Job drawing, mm, ordinate dimensions from the low corner. One solid piece. A direction names the side the tool comes from. Give positions to 0.01 mm unless a question says otherwise; leave off trailing zeros. Loops run counter-clockwise (first coordinate to the right, second up) from the corner with the lowest first, then second, coordinate; pieces in that order, holes last. Notation, with made-up numbers: (42, -26.5) - (70, -26.5) arc R15 ccw to (70, -1.5) - close; hole circle Ø1 at (26.5, 35). An arc over 180 degrees is marked (long way). Answer as CSV lines item,"result". Start each with the question number.
Item 1: Saw through at D-D on x = 18. Give the cut face in (y, z).
Item 2: Saw through at A-A on x = 120. Give the cut face in (y, z).
Item 3: Tool access for the marked faces 1, 2 and 3: list every direction of +Z, -Z, +X, -X, +Y, -Y with a clear straight run to the whole face (end or side of a thin tool).
Item 4: Drill centre lines: L1, parallel to Y at x = 120, z = 38.5; L2, parallel to Y at x = 120, z = 33.5; L3, parallel to Z at x = 220, y = 138. Where is each one in solid material? Low to high. Write a range as from..to.
Item 5: Pin check, flat tips, straight feed: pin 1 (12 mm diameter, centred on y = 66, z = 12.5, fed in from -X); pin 2 (4 mm diameter, centred on y = 175.5, z = 40.5, fed in from +X); pin 3 (2 mm diameter, centred on x = 121.5, y = 207, fed in from +Z). Stop position of each tip, or through.
Item 6: Pull direction Y, two halves, no side cores. Call the marked faces 4, 5 and 6: pulls with the +Y half, pulls with the -Y half, needs draft (parallel to the pull), parting line crosses it, or undercut.
Item 7: Saw through at B-B on y = 120. Give the cut face in (x, z), plus the area to 3 significant figures.
Item 8: Saw through at C-C on z = 39. Give the cut face in (x, y).
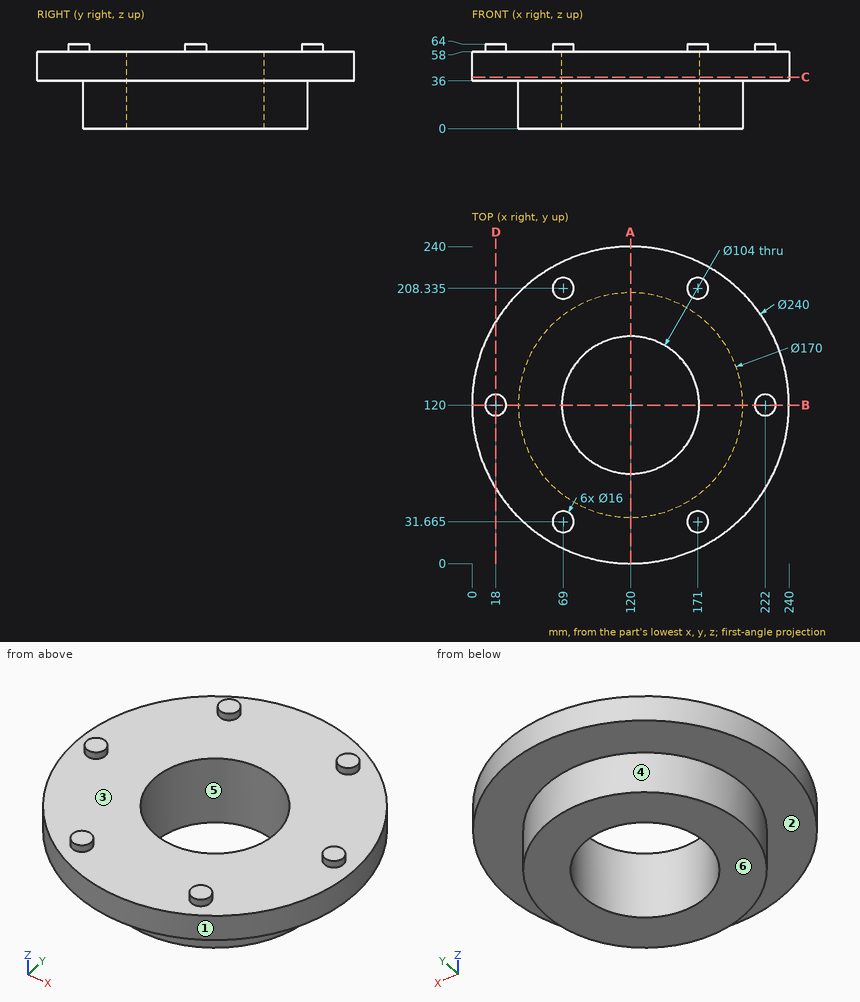
Responses:
1,outline,"(56.79, 36) - (183.21, 36) - (183.21, 58) - (128, 58) - (128, 64) - (112, 64) - (112, 58) - (56.79, 58) - close"
2,outline,"(0, 36) - (35, 36) - (35, 0) - (68, 0) - (68, 58) - (0, 58) - close; (172, 0) - (205, 0) - (205, 36) - (240, 36) - (240, 58) - (172, 58) - close"
3,face 1,"+Z, -Z"
3,face 2,"-Z"
3,face 3,"+Z"
4,L1,"0..68, 172..240"
4,L2,"35..68, 172..205"
4,L3,"36..58"
5,pin 1,"x = 49.85"
5,pin 2,"x = 227.41"
5,pin 3,"z = 58"
6,face 4,"parting line crosses it"
6,face 5,"undercut"
6,face 6,"needs draft"
7,outline,"(0, 36) - (35, 36) - (35, 0) - (68, 0) - (68, 58) - (26, 58) - (26, 64) - (10, 64) - (10, 58) - (0, 58) - close; (172, 0) - (205, 0) - (205, 36) - (240, 36) - (240, 58) - (230, 58) - (230, 64) - (214, 64) - (214, 58) - (172, 58) - close"
7,area,"5,560 mm2"
8,outline,"circle Ø240 at (120, 120); hole circle Ø104 at (120, 120)"
